Geometry check sheet. Reference: drawing and pictorial views, mm from the part's lowest x, y, z. Coordinates: 2 decimals unless noted, no trailing zeros. Loops run counter-clockwise (first coordinate to the right, second up) from the corner with the lowest first, then second, coordinate; pieces in that order, holes last. Notation, with made-up numbers: (64, 13) - (105, 13) arc R27 cw to (105, 33) - close; hole circle Ø10 at (29.5, 59). An arc over 180 degrees is marked (long way). One line per item, written item: value.
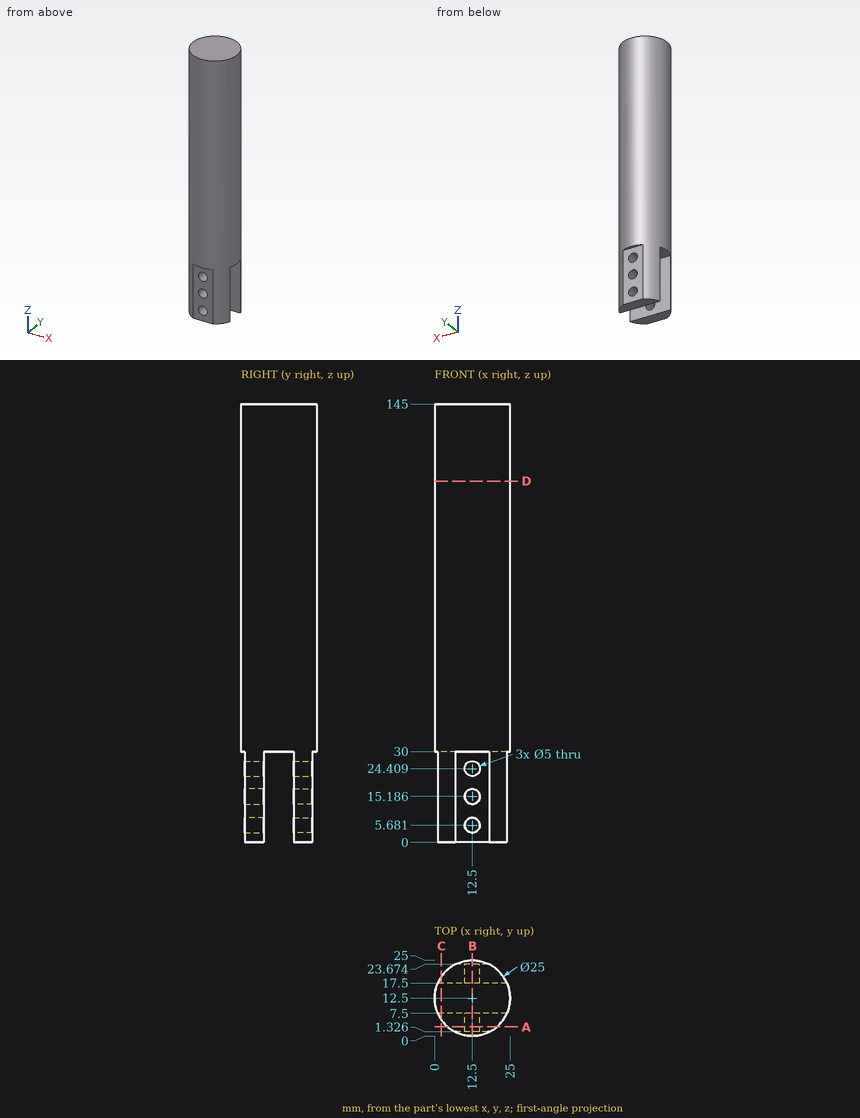
(1) Cross-section at C-C on x = 2.25. Record the cut outline in (y, z) (1 decimal), and give its area (4 significant figures).
Reply:
outline: (5.3, 0) - (7.5, 0) - (7.5, 30) - (17.5, 30) - (17.5, 0) - (19.7, 0) - (19.7, 145) - (5.3, 145) - close
area: 1,775 mm2
(2) Go/stop test with flat-tipped pins: pin 1 Ø8 at (x, z) = (12.5, 15.19) entering from -Y; pin 2 Ø8 at (y, z) = (19, 98) entering from -X; pin 3 Ø6 at (y, z) = (9.5, 39.5) entering from -X; pin 4 Ø1.5 at (x, z) = (4.5, 121) entering from -Y. Record where each tip stops, or that it passes through.
Reply:
pin 1: y = 1.33
pin 2: x = 0.25
pin 3: x = 0
pin 4: y = 2.32
(3) Cross-section at D-D on z = 119.5. Record the cut outline in (x, y), and give its area (3 significant figures).
Reply:
outline: circle Ø25 at (12.5, 12.5)
area: 491 mm2
(4) Cross-section at B-B on x = 12.5. State how many separate pieces and enclosed holes the cut face has, and give its area (3 significant figures).
Reply:
separate pieces: 7
enclosed holes: 0
area: 3,060 mm2
(5) Material ranges on probe 1 along Z at (x, y) = (12.25, 3.75); probe 2 along Y at (x, z) = (15.5, 21.5); probe 3 along Y at (x, z) = (12.25, 99), recorded low to high. Write a range as from..to.
Reply:
probe 1: 0..3.19, 8.17..12.7, 17.67..21.92, 26.9..145
probe 2: 1.33..7.5, 17.5..23.67
probe 3: 0..25
(6) Cross-section at A-A on y = 3. Record the cut outline in (x, z).
Reply:
outline: (4.38, 0) - (20.62, 0) - (20.62, 145) - (4.38, 145) - close; hole circle Ø5 at (12.5, 5.68); hole circle Ø5 at (12.5, 15.19); hole circle Ø5 at (12.5, 24.41)
